The model under review builds one solid part; all positions refer to its coordinate system, in mm. Face numbers are marked on the shaded views. A direction names the side the tool comes from. Coordinates: 2 decimals unless noted, no trailing zeros. One line per item, written item: value.
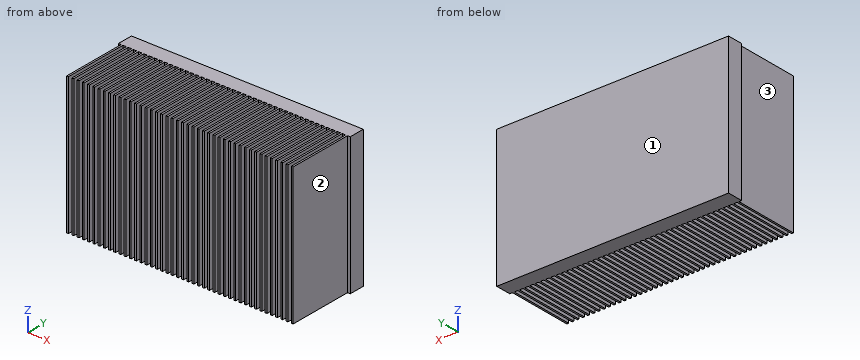
```python
from build123d import *

# Parameters (mm, degrees)
SKETCH_1_W      = 253
SKETCH_1_H      = 17
SKETCH_1_W_2    = 2
SKETCH_1_H_2    = 71
EXTRUDE_1_DEPTH = 150


with BuildPart() as part:
    # 草图1 → 凸台-拉伸1 (new body)
    with BuildSketch(Plane.XY):
        with Locations((126.5, -8.5)):
            Rectangle(SKETCH_1_W, SKETCH_1_H)
        with Locations((3.9, -52.5)):
            Rectangle(SKETCH_1_W_2, SKETCH_1_H_2)
        with Locations((9.6, -52.5)):
            Rectangle(SKETCH_1_W_2, SKETCH_1_H_2)
        with Locations((15.3, -52.5)):
            Rectangle(SKETCH_1_W_2, SKETCH_1_H_2)
        with Locations((21, -52.5)):
            Rectangle(SKETCH_1_W_2, SKETCH_1_H_2)
        with Locations((26.7, -52.5)):
            Rectangle(SKETCH_1_W_2, SKETCH_1_H_2)
        with Locations((32.4, -52.5)):
            Rectangle(SKETCH_1_W_2, SKETCH_1_H_2)
        with Locations((38.1, -52.5)):
            Rectangle(SKETCH_1_W_2, SKETCH_1_H_2)
        with Locations((43.8, -52.5)):
            Rectangle(SKETCH_1_W_2, SKETCH_1_H_2)
        with Locations((49.5, -52.5)):
            Rectangle(SKETCH_1_W_2, SKETCH_1_H_2)
        with Locations((55.2, -52.5)):
            Rectangle(SKETCH_1_W_2, SKETCH_1_H_2)
        with Locations((60.9, -52.5)):
            Rectangle(SKETCH_1_W_2, SKETCH_1_H_2)
        with Locations((66.6, -52.5)):
            Rectangle(SKETCH_1_W_2, SKETCH_1_H_2)
        with Locations((72.3, -52.5)):
            Rectangle(SKETCH_1_W_2, SKETCH_1_H_2)
        with Locations((78, -52.5)):
            Rectangle(SKETCH_1_W_2, SKETCH_1_H_2)
        with Locations((83.7, -52.5)):
            Rectangle(SKETCH_1_W_2, SKETCH_1_H_2)
        with Locations((89.4, -52.5)):
            Rectangle(SKETCH_1_W_2, SKETCH_1_H_2)
        with Locations((95.1, -52.5)):
            Rectangle(SKETCH_1_W_2, SKETCH_1_H_2)
        with Locations((100.8, -52.5)):
            Rectangle(SKETCH_1_W_2, SKETCH_1_H_2)
        with Locations((106.5, -52.5)):
            Rectangle(SKETCH_1_W_2, SKETCH_1_H_2)
        with Locations((112.2, -52.5)):
            Rectangle(SKETCH_1_W_2, SKETCH_1_H_2)
        with Locations((117.9, -52.5)):
            Rectangle(SKETCH_1_W_2, SKETCH_1_H_2)
        with Locations((123.6, -52.5)):
            Rectangle(SKETCH_1_W_2, SKETCH_1_H_2)
        with Locations((129.3, -52.5)):
            Rectangle(SKETCH_1_W_2, SKETCH_1_H_2)
        with Locations((135, -52.5)):
            Rectangle(SKETCH_1_W_2, SKETCH_1_H_2)
        with Locations((140.7, -52.5)):
            Rectangle(SKETCH_1_W_2, SKETCH_1_H_2)
        with Locations((146.4, -52.5)):
            Rectangle(SKETCH_1_W_2, SKETCH_1_H_2)
        with Locations((152.1, -52.5)):
            Rectangle(SKETCH_1_W_2, SKETCH_1_H_2)
        with Locations((157.8, -52.5)):
            Rectangle(SKETCH_1_W_2, SKETCH_1_H_2)
        with Locations((163.5, -52.5)):
            Rectangle(SKETCH_1_W_2, SKETCH_1_H_2)
        with Locations((169.2, -52.5)):
            Rectangle(SKETCH_1_W_2, SKETCH_1_H_2)
        with Locations((174.9, -52.5)):
            Rectangle(SKETCH_1_W_2, SKETCH_1_H_2)
        with Locations((180.6, -52.5)):
            Rectangle(SKETCH_1_W_2, SKETCH_1_H_2)
        with Locations((186.3, -52.5)):
            Rectangle(SKETCH_1_W_2, SKETCH_1_H_2)
        with Locations((192, -52.5)):
            Rectangle(SKETCH_1_W_2, SKETCH_1_H_2)
        with Locations((197.7, -52.5)):
            Rectangle(SKETCH_1_W_2, SKETCH_1_H_2)
        with Locations((203.4, -52.5)):
            Rectangle(SKETCH_1_W_2, SKETCH_1_H_2)
        with Locations((209.1, -52.5)):
            Rectangle(SKETCH_1_W_2, SKETCH_1_H_2)
        with Locations((214.8, -52.5)):
            Rectangle(SKETCH_1_W_2, SKETCH_1_H_2)
        with Locations((220.5, -52.5)):
            Rectangle(SKETCH_1_W_2, SKETCH_1_H_2)
        with Locations((226.2, -52.5)):
            Rectangle(SKETCH_1_W_2, SKETCH_1_H_2)
        with Locations((231.9, -52.5)):
            Rectangle(SKETCH_1_W_2, SKETCH_1_H_2)
        with Locations((237.6, -52.5)):
            Rectangle(SKETCH_1_W_2, SKETCH_1_H_2)
        with Locations((243.3, -52.5)):
            Rectangle(SKETCH_1_W_2, SKETCH_1_H_2)
        with Locations((249, -52.5)):
            Rectangle(SKETCH_1_W_2, SKETCH_1_H_2)
    extrude(amount=EXTRUDE_1_DEPTH)


solid = part.part
```
(1) Add section A-A on y = -68. State how many separate pieces and enclosed holes the cut face has, then the cut area to 3 significant figures.
Checks:
separate pieces: 44
enclosed holes: 0
area: 13,200 mm^2
(2) Tool access review of the marked faces 1, 2 and 3: name each direction out of +Z, -Z, +X, -X, +Y, -Y from which nothing blocks a thin tool from reaching the whole face with its end or side.
Checks:
face 1: +Z, -Z, +X, -X, +Y
face 2: +Z, -Z, +X, -Y
face 3: +Z, -Z, -X, -Y
(3) To check wall thickness, follow L1, parallel to Y at x = 216.5, z = 10. State the ranges of the line that lie inside material, in increasing order. Write a range as [from, to].
Checks:
L1: [-17, 0]
(4) Insertion check: pin 1 Ø1.9 at (x, z) = (17.5, 76.5) entering from -Y; pin 2 Ø21.5 at (y, z) = (-69, 79) entering from +X; pin 3 Ø21.5 at (y, z) = (-52.5, 80) entering from -X. Each pin has a flat end and moves straight along its axis. Give the tip position at first contact, or say it passes through.
Checks:
pin 1: y = -17
pin 2: x = 250
pin 3: x = 2.9
